Geometry check sheet. Reference: drawing and pictorial views, mm from the part's lowest x, y, z. A direction names the side the tool comes from. Coordinates: 2 decimals unless noted, no trailing zeros. Write each loop counter-clockwise with the first axis right and the second up, starting at its lowest first coordinate (ties: lowest second). Pieces come first, ordered by that corner, then holes. Notation, with made-up numbers: (19, 40.25) -> (32, 40.25) arc R6 ccw to (32, 46.25) -> close; hole circle Ø11 at (38.5, 54.25). An arc over 180 degrees is marked (long way). Answer in a Markdown table with one row per item.
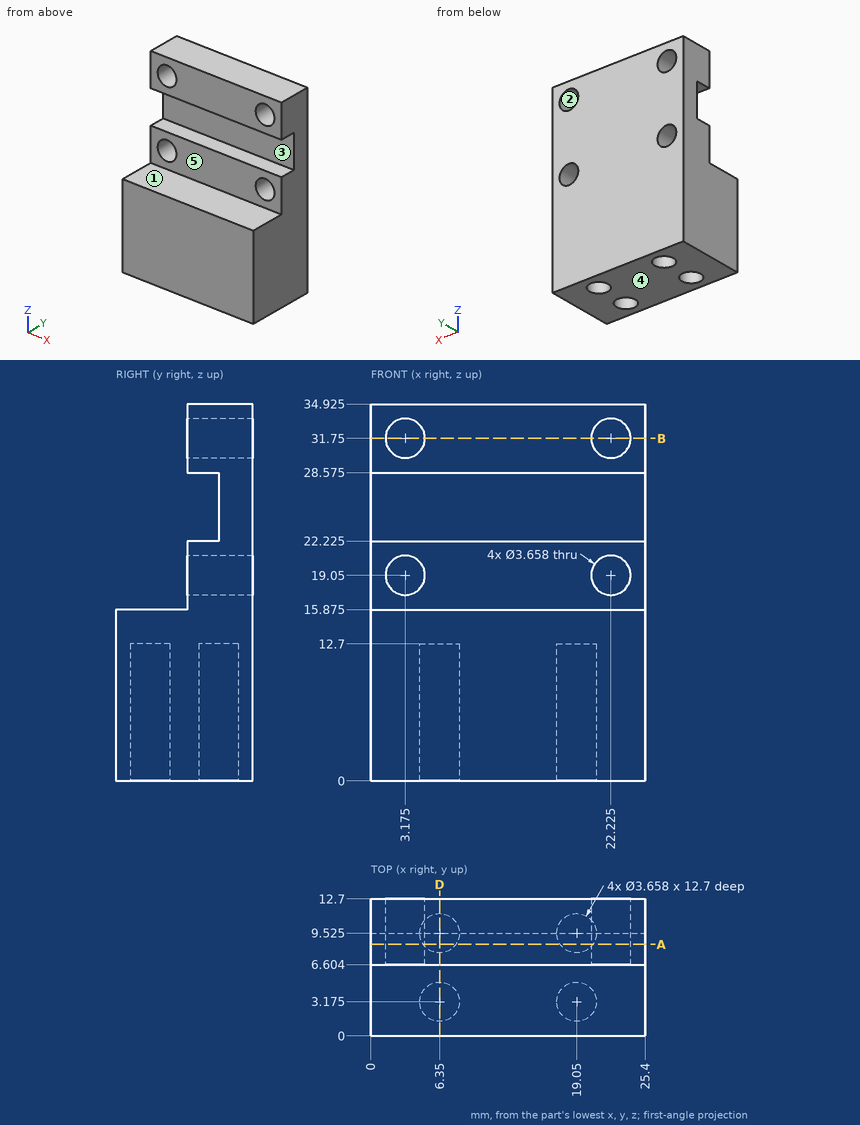
1. Thickness scan on line 1 (Y direction, x = 6.35, z = 2.5); line 2 (Z direction, x = 17.75, y = 7.25) (1 decimal); line 3 (Z direction, x = 6.25, y = 9.25) (1 decimal). Record the ranges inside material, lowest first. Write a range as from..to.
Geometry says:
| item | result |
|---|---|
| line 1 | 0..1.35, 5..7.7, 11.35..12.7 |
| line 2 | 0..22.2, 28.6..34.9 |
| line 3 | 12.7..22.2, 28.6..34.9 |
2. Depth check by flat-ended pin: P1, Ø1.9, axis at x = 14.5, z = 26.5, coming from the -Y side (3 decimals); P2, Ø2, axis at x = 14.5, y = 1.5, coming from the -Z side; P3, Ø1.9, axis at x = 17.5, z = 20.5, coming from the -Y side; P4, Ø2, axis at x = 7, y = 2.5, coming from the +Z side (3 decimals). Enter the tip coordinate at first touch or a pass-through.
Geometry says:
| item | result |
|---|---|
| P1 | y = 9.525 |
| P2 | z = 0 |
| P3 | y = 6.6 |
| P4 | z = 15.875 |
3. Section check B-B, the plane z = 31.75. Record the boundary of the cut face in (x, y), plus the area to 3 significant figures.
Geometry says:
| item | result |
|---|---|
| outline | (0, 6.6) -> (1.35, 6.6) -> (1.35, 12.7) -> (0, 12.7) -> close; (5, 6.6) -> (20.4, 6.6) -> (20.4, 12.7) -> (5, 12.7) -> close; (24.05, 6.6) -> (25.4, 6.6) -> (25.4, 12.7) -> (24.05, 12.7) -> close |
| area | 110 mm^2 |
4. Mould release check, pull along Z, two halves, no side actions. Record for the marked faces 3, 4 and 5: released by +Z, released by -Z, zero draft, split by the parting line, or undercut.
Geometry says:
| item | result |
|---|---|
| face 3 | undercut |
| face 4 | released by -Z |
| face 5 | zero draft |
5. Tool access check on the marked faces 1 and 2. Record the directions out of +Z, -Z, +X, -X, +Y, -Y that give a thin tool (end or side, any length) a straight path to the whole face; none if there is none.
Geometry says:
| item | result |
|---|---|
| face 1 | +Z, +X, -X, -Y |
| face 2 | +Y, -Y |
6. Section check A-A, the plane y = 8.5. State how many separate pieces and enclosed holes the cut face has, plus the area to 3 significant figures.
Geometry says:
| item | result |
|---|---|
| separate pieces | 2 |
| enclosed holes | 4 |
| area | 607 mm^2 |
7. Section check D-D, the plane x = 6.35. Record the boundary of the cut face in (y, z) (1 decimal).
Geometry says:
| item | result |
|---|---|
| outline | (0, 0) -> (1.3, 0) -> (1.3, 12.7) -> (5, 12.7) -> (5, 0) -> (7.7, 0) -> (7.7, 12.7) -> (11.4, 12.7) -> (11.4, 0) -> (12.7, 0) -> (12.7, 34.9) -> (6.6, 34.9) -> (6.6, 28.6) -> (9.5, 28.6) -> (9.5, 22.2) -> (6.6, 22.2) -> (6.6, 15.9) -> (0, 15.9) -> close |
